Geometry check sheet. Reference: drawing and pictorial views, mm from the part's lowest x, y, z. Coordinates: 2 decimals unless noted, no trailing zeros. Loops run counter-clockwise (first coordinate to the right, second up) from the corner with the lowest first, then second, coordinate; pieces in that order, holes last.
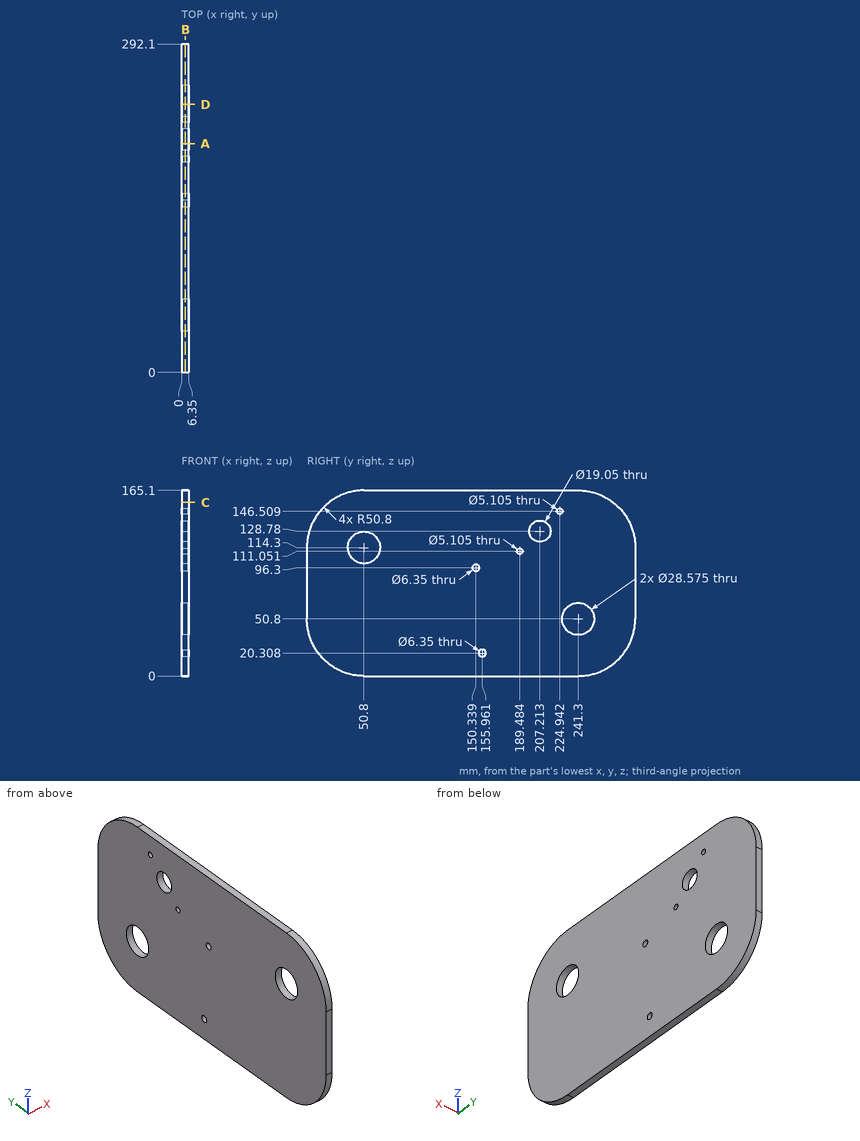
1) Depth check by flat-ended pin: pin 1 (5 mm diameter, centred on y = 155.96, z = 20.31, fed in from +X). Enter the tip coordinate at first touch or a pass-through.
Data:
pin 1: passes through
2) Material ranges on probe 1 along Z at (x, y) = (3.5, 206.5); probe 2 along Y at (x, z) = (2.25, 111.5); probe 3 along Y at (x, z) = (6, 120) (1 decimal), recorded low to high.
Data:
probe 1: z = 0 to 119.28, 138.28 to 165.1
probe 2: y = 0 to 36.79, 64.81 to 186.97, 192 to 292.1
probe 3: y = 0.3 to 37.7, 63.9 to 203.5, 210.9 to 291.8
3) Section check A-A on y = 203.5. Record the cut outline in (x, z), and give its area (3 significant figures).
Data:
outline: (0, 0) - (6.35, 0) - (6.35, 120.01) - (0, 120.01) - close; (0, 137.55) - (6.35, 137.55) - (6.35, 165.1) - (0, 165.1) - close
area: 937 mm2
4) Section check B-B on x = 3.25. Count the separate pieces of the cut face and the enclosed holes in it, and give its area (3 significant figures).
Data:
separate pieces: 1
enclosed holes: 7
area: 44,300 mm2
5) Section check C-C on z = 154.5. Record the cut outline in (x, y).
Data:
outline: (0, 19.74) - (6.35, 19.74) - (6.35, 272.36) - (0, 272.36) - close
6) Section check D-D on y = 238.5. Record the cut outline in (x, z).
Data:
outline: (0, 0) - (6.35, 0) - (6.35, 36.79) - (0, 36.79) - close; (0, 64.81) - (6.35, 64.81) - (6.35, 165.1) - (0, 165.1) - close
